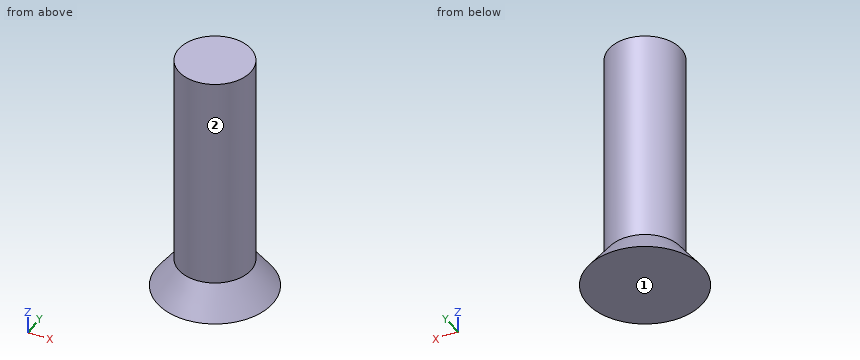
from build123d import *

# Parameters (mm, degrees)
SKETCH1_R           = 4
BOSS_EXTRUDE1_DEPTH = 2
SKETCH2_R           = 2.5
BOSS_EXTRUDE2_DEPTH = 15


with BuildPart() as part:
    # Sketch1 → Boss-Extrude1 (new body)
    with BuildSketch(Plane(origin=(0, 0, 0), x_dir=(0, 1, 0), z_dir=(0, 0, 1))):
        with Locations(Location((0, 0, 0), (0, 0, 270))):
            Circle(SKETCH1_R)
    extrude(amount=BOSS_EXTRUDE1_DEPTH)

    # Sketch2 → Boss-Extrude2 (add)
    with BuildSketch(Plane.XY.offset(2)):
        Circle(SKETCH2_R)
    extrude(amount=BOSS_EXTRUDE2_DEPTH)

    # Sketch3 → Cut-Revolve1 (revolve, cut)
    with BuildSketch(Plane.YZ, mode=Mode.PRIVATE) as cut_revolve1_sk:
        Polygon((-2.5, 2), (-4, 2), (-4, 0), align=None)
    revolve(cut_revolve1_sk.sketch.rotate(Axis((0, 0, 0), (0, 0, 1)), 270), axis=Axis((0, 0, 0), (0, 0, 1)), mode=Mode.SUBTRACT)


solid = part.part
Input: part model. Units: mm. Frame: model coordinates. Face numbers are marked on the shaded views. A direction names the side the tool comes from. Round coordinates to 2 decimals unless told otherwise and drop trailing zeros. Loops run counter-clockwise (first coordinate to the right, second up) from the corner with the lowest first, then second, coordinate; pieces in that order, holes last. Notation, with made-up numbers: M 72,54.5 L 98,54.5 A15 ccw 98,67.5 Z; hole C 10,84 d1. An arc over 180 degrees is marked long. Answer as CSV lines item,"result". Start each with the question number.
(1) Reachability of the marked faces 1 and 2 from +Z, -Z, +X, -X, +Y, -Y: full face, straight path, thin tool, end or side. Return the list, or none.
(2) Section D-D, the plane z = 12. Output: boundary loops of the cut face in (x, y).
(3) First-contact query: pin 1 (4 mm diameter, centred on y = -1, z = 4, fed in from +X); pin 2 (1.5 mm diameter, centred on x = 1.5, z = 2.5, fed in from -Y). Flat tips, straight axial feed; report the tip coordinate or a pass-through.
(4) Line query: line 1 (Y direction, x = 0, z = 11.75); line 2 (X direction, y = 1, z = 11.75); line 3 (X direction, y = -1.5, z = 15). Output: solid intervals per line, ascending. Write a range as [from, to].
(5) Section C-C, the plane z = 1. Output: boundary loops of the cut face in (x, y), plus the area to 3 significant figures.
(6) Section A-A, the plane y = 0. Output: boundary loops of the cut face in (x, z).
Values found:
1,face 1,"-Z, +X, -X, +Y, -Y"
1,face 2,"+Z"
2,outline,"C 0,0 d5"
3,pin 1,"stops at x = 2.5"
3,pin 2,"stops at y = -2.38"
4,line 1,"y = [-2.5, 2.5]"
4,line 2,"x = [-2.29, 2.29]"
4,line 3,"x = [-2, 2]"
5,outline,"C 0,0 d6.5"
5,area,"33.2 mm²"
6,outline,"M -4,0 L 4,0 L 2.5,2 L 2.5,17 L -2.5,17 L -2.5,2 Z"
